Input: part model. Units: mm. Frame: model coordinates. A direction names the side the tool comes from. Give positions to 0.01 mm unless a question says otherwise; leave off trailing zeros. Loops run counter-clockwise (first coordinate to the right, second up) from the corner with the lowest first, then second, coordinate; pieces in that order, holes last. Notation, with made-up numbers: (37.5, 76) -> (69.5, 76) arc R34 ccw to (69.5, 108) -> close; hole circle Ø9 at (63, 62.25). An arc over 180 degrees is marked (long way). Answer as a JSON object with one key per item and string values.
Autodesk Inventor part; units mm, degrees
ref_plane "YZ Plane" through (0, 0, 0) normal (1, 0, 0) x (0, 1, 0)
ref_plane "XZ Plane" through (0, 0, 0) normal (0, 1, 0) x (-1, 0, 0)
ref_plane "XY Plane" through (0, 0, 0) normal (0, 0, 1) x (1, 0, 0)
sketch "Sketch1" plane through (0, 0, 0) normal (0, 1, 0) x (-1, 0, 0)
  line L0 (0, 0) -> (-50, 0)
  line L1 (-50, 0) -> (-50, -30)
  line L2 (-50, -30) -> (0, -30)
  line L3 (0, -30) -> (0, 0)
  dimension "d0" = 50
  dimension "d1" = 30
extrude "Extrusion1" add sketch "Sketch1" along normal blind 3
sketch "Sketch2" plane through (0, 3, 0) normal (0, 1, 0) x (1, 0, 0)
  circle A0 centre (15, 15) radius 8.8
  line L0 (0, 30) -> (0, 0)
  line L1 (0, 0) -> (50, 0)
  circle A1 centre (38, 15) radius 8.8
  dimension "d4" = 17.6
  dimension "d5" = 15
  dimension "d6" = 15
  dimension "d12" = 17.6
  dimension "d16" = 0
  dimension "d17" = 23
extrude "Extrusion2" cut sketch "Sketch2" against normal blind 1
sketch "Sketch3" plane through (15, 2, -15) normal (0, 1, 0) x (1, 0, 0)
  circle A0 centre (0, 0) radius 6.9
  circle A1 centre (23, 0) radius 6.9
  circle A2 centre (23, 0) radius 8.8
  point P0 (-15, -15)
  point P1 (-13.4125, -13.4125)
  dimension "d9" = 13.8
  dimension "d13" = 13.8
  dimension "d14" = 0
  dimension "d15" = 0
extrude "Extrusion3" cut sketch "Sketch3" against normal through all contours A0 | A1
properties part number "Proto_Valve_Fitting_TestPlate"
Q1. Pin query (flat end, axial travel): pin 1 (3 mm diameter, centred on x = 37, z = -7, fed in from +Y); pin 2 (14 mm diameter, centred on x = 38, z = -13.5, fed in from +Y). Return the tip coordinate at first contact, or that it passes through.
Evaluation:
{"pin 1": "stops at y = 3", "pin 2": "stops at y = 2"}
Q2. Access query for faces 5 (the flat face through (10, 2, -10)), 6 (the cylindrical face through (18.184, 1.014, -8.879)). Directions: +Z, -Z, +X, -X, +Y, -Y. A direction counts if a zero-diameter tool reaches every point of the face in a straight line with its end or side. Return the directions, or none.
Evaluation:
{"face 5": "+Y", "face 6": "+Y, -Y"}
Q3. Section C-C, the plane y = 1.5. Return the cut outline in (x, z).
Evaluation:
{"outline": "(0, -30) -> (50, -30) -> (50, 0) -> (0, 0) -> close; hole circle Ø13.8 at (15, -15); hole circle Ø13.8 at (38, -15)"}
Q4. Draft query along Z for faces 1 (the flat face through (25, 1, -30)), 2 (the flat face through (25, 1, 0)), 3 (the cylindrical face through (32.524, 1.014, -10.801)), 4 (the flat face through (25, 3, -15)). Return one class per face: +Z half, -Z half, draft (parallel to the pull), parting line (faces both ways), or undercut.
Evaluation:
{"face 1": "-Z half", "face 2": "+Z half", "face 3": "undercut", "face 4": "draft"}
Q5. Section D-D, the plane x = 13.5. Return the cut outline in (y, z).
Evaluation:
{"outline": "(0, -30) -> (3, -30) -> (3, -23.67) -> (2, -23.67) -> (2, -21.73) -> (0, -21.73) -> close; (0, -8.27) -> (2, -8.27) -> (2, -6.33) -> (3, -6.33) -> (3, 0) -> (0, 0) -> close"}
Q6. Section A-A, the plane z = -15. Return the cut outline in (x, y).
Evaluation:
{"outline": "(0, 0) -> (8.1, 0) -> (8.1, 2) -> (6.2, 2) -> (6.2, 3) -> (0, 3) -> close; (21.9, 0) -> (31.1, 0) -> (31.1, 2) -> (29.2, 2) -> (29.2, 3) -> (23.8, 3) -> (23.8, 2) -> (21.9, 2) -> close; (44.9, 0) -> (50, 0) -> (50, 3) -> (46.8, 3) -> (46.8, 2) -> (44.9, 2) -> close"}
Q7. Section B-B, the plane x = 38. Return the cut outline in (y, z), then the cut area to 3 significant figures.
Evaluation:
{"outline": "(0, -30) -> (3, -30) -> (3, -23.8) -> (2, -23.8) -> (2, -21.9) -> (0, -21.9) -> close; (0, -8.1) -> (2, -8.1) -> (2, -6.2) -> (3, -6.2) -> (3, 0) -> (0, 0) -> close", "area": "44.8 mm2"}
Q8. Ray query, line 1 along X through (y, z) = (2.7, -15); line 2 along X through (y, z) = (1.4, -15); line 3 along Z through (x, y) = (15, 2.35). Return the intervals inside material, ascending.
Evaluation:
{"line 1": "x = 0 to 6.2, 23.8 to 29.2, 46.8 to 50", "line 2": "x = 0 to 8.1, 21.9 to 31.1, 44.9 to 50", "line 3": "z = -30 to -23.8, -6.2 to 0"}
